The model under review builds one solid part; all positions refer to its coordinate system, in mm. A direction names the side the tool comes from. Round coordinates to 2 decimals unless told otherwise and drop trailing zeros. Write each loop counter-clockwise with the first axis right and the second up, starting at its lowest first coordinate (ties: lowest second). Pieces come first, ordered by that corner, then holes. Notation, with made-up numbers: M 66,49 L 85,49 A20 cw 85,83 Z; hole C 33,19.5 d8. An arc over 180 degrees is marked long. Write item = value, one per line. Start each with the question number.
Item 1: For pin 1 Ø3 at (y, z) = (16.02, 18.75) entering from +X; pin 2 Ø4 at (x, y) = (6, 7) entering from +Z; pin 3 Ø2 at (y, z) = (15, 16.5) entering from -X; pin 4 Ø7 at (x, z) = (10, 2) entering from +Y, all flat-tipped, find the tip position at first contact; note any pin that passes through.
Item 2: Take a section at D-D, the plane x = -10. Give the boundary of the cut face in (y, z), plus the area to 3 significant figures.
Item 3: Tool access review of faces 1 (the flat face through (7, -13.5, 2)), 2 (the flat face through (7, 13.5, 2)), 3 (the flat face through (0, 0, 3)): name each direction out of +Z, -Z, +X, -X, +Y, -Y from which nothing blocks a thin tool from reaching the whole face with its end or side.
Item 4: Take a section at A-A, the plane y = 0. Give the boundary of the cut face in (x, z), plus the area to 3 significant figures.
Item 5: To check wall thickness, follow line 1 along Y through (x, z) = (5, 2); line 2 along Y through (x, z) = (19.4, 18.75); line 3 along Z through (x, y) = (4.5, -4). State the ranges of each line that lie inside material, in increasing order.
Item 6: Take a section at C-C, the plane z = 28. Give the boundary of the cut face in (x, y).
Item 7: Take a section at B-B, the plane x = 5. Give the boundary of the cut face in (y, z).
Item 8: The part is to be moulded in two halves that separate along X. For faces 4 (the cylindrical face through (6.2, -8.04, 1.52)), 5 (the cylindrical face through (-11.789, -11.696, 1.521)), 6 (the cylindrical face through (19.02, 0.71, 49.99)), say which applies: +X half, -X half, draft (parallel to the pull), parting line (faces both ways), or undercut.
Autodesk Inventor part; units mm, degrees
ref_plane "YZ Plane" through (0, 0, 0) normal (1, 0, 0) x (0, 1, 0)
ref_plane "XZ Plane" through (0, 0, 0) normal (0, 1, 0) x (-1, 0, 0)
ref_plane "XY Plane" through (0, 0, 0) normal (0, 0, 1) x (1, 0, 0)
sketch "スケッチ1" plane through (0, 0, 0) normal (0, 0, 1) x (1, 0, 0)
  circle A0 centre (0, 0) radius 13.5
  line L0 (0, 13.5) -> (14.5, 13.5)
  line L1 (14.5, 13.5) -> (14.5, -13.5)
  line L2 (14.5, -13.5) -> (0, -13.5)
  line L3 (0, -13.5) -> (0, 13.5)
  line L4 (0, 0) -> (14.5, 0) construction
  point P0 (0, 13.5)
  point P1 (0, -13.5)
  point P2 (0, -13.5)
  dimension "d0" = 27
  dimension "d1" = 27
  dimension "d2" = 14.5
extrude "プレート1" add sketch "スケッチ1" along normal blind 3
sketch "スケッチ2" plane through (17.5, 13.5, 6) normal (1, 0, 0) x (0, 1, 0)
  line L0 (-27, 0) -> (0, 0)
  line L1 (0, 0) -> (0, 19)
  line L2 (0, 19) -> (-27, 19)
  line L3 (-27, 19) -> (-27, 0)
edge flange "フランジ1" height 25 angle 90 thickness 3 bend radius 3 thickness toward (1, 0, 0) relief tear relief width 3 relief depth 1.5 edges at (14.5, 0, 3) wall of the first edge with corners at (17.5, -13.5, 6) (17.5, 13.5, 6) (17.5, 13.5, 25) (17.5, -13.5, 25)
bend "曲げ1"
corner "コーナー1"
sketch "スケッチ3" plane through (0, 0, 0) normal (0, 0, -1) x (-1, 0, 0)
  point P0 (0, 0)
  point P1 (10, 0)
  point P2 (-5, 8.6603)
  point P3 (-5, -8.6603)
  dimension "d14" = 10
  dimension "d17" = 360
hole "穴1" at (-10, 0, 0) at (5, 8.6603, 0) at (5, -8.6603, 0) direction (0, 0, 1) diameter 2.7 depth 3
sketch "スケッチ4" plane through (20.5, -13.5, 25) normal (1, 0, 0) x (0, 0, -1)
  circle A0 centre (-3, 13.5) radius 22
  line L0 (25, 27) -> (25, 0)
  line L1 (0, 27) -> (19, 27)
  point P0 (25, 13.5)
  dimension "d26" = 44
  dimension "d29" = 28
  dimension "d46" = 13.5
extrude "押し出し1" add sketch "スケッチ4" against normal up to surface (3 mm away)
sketch "スケッチ5" plane through (20.5, -13.5, 6) normal (1, 0, 0) x (0, 0, -1)
  arc A0 (-4.629, 27) -> (-4.629, 0) centre (-22, 13.5) ccw
  circle A1 centre (-22, 13.5) radius 14.5
  point P0 (6, 13.5)
  dimension "d30" = 29
extrude "押し出し2" cut sketch "スケッチ5" against normal up to surface (3 mm away)
sketch "スケッチ6" plane through (20.5, 0, 28) normal (1, 0, 0) x (0, 0, 1)
  point P0 (-28, 0)
sketch "スケッチ7" plane through (20.5, -13.5, 6) normal (1, 0, 0) x (0, 0, -1)
  circle A0 centre (-22, 13.5) radius 14.5
  point P0 (6, 13.5)
  point P1 (-40.5, 13.5)
  point P2 (-12.75, -2.5215)
  point P3 (-12.75, 29.5215)
  dimension "d33" = 18.5
  dimension "d36" = 360
hole "穴2" at (20.5, 0, 46.5) at (20.5, -16.0215, 18.75) at (20.5, 16.0215, 18.75) direction (-1, 0, 0) diameter 2.7 depth 3
fillet "フィレット1" radius 10 2 edges at (19, -13.5, 10.629) (19, 13.5, 10.629)
sketch "スケッチ8" plane through (0, 0, 0) normal (0, 0, -1) x (-1, 0, 0)
  line L0 (0, 13.5) -> (-14.5, 13.5)
  line L1 (0, 13.5) -> (13.5, 13.5)
  line L2 (13.5, 13.5) -> (13.5, -13.5)
  line L3 (13.5, -13.5) -> (0, -13.5)
  line L4 (0, -13.5) -> (0, 13.5)
  circle A0 centre (-5, -8.6603) radius 1.35
  circle A1 centre (-5, 8.6603) radius 1.35
  circle A2 centre (10, 0) radius 1.35
  line L5 (0, 13.5) -> (-14.5, 13.5)
  line L6 (-14.5, 13.5) -> (-14.5, -13.5)
  line L7 (-14.5, -13.5) -> (0, -13.5)
  arc A3 (0, -13.5) -> (0, 13.5) centre (0, 0) ccw
  point P0 (13.5, 0)
  dimension "d47" = 13.5
  dimension "d48" = 27
extrude "押し出し3" add sketch "スケッチ8" against normal up to surface (3 mm away) contours L1 L2 A3 | A3 L2 L3
fillet "フィレット2" radius 6 2 edges at (-13.5, 13.5, 1.5) (-13.5, -13.5, 1.5)
equation "\"d24\" = Thickness"
equation "\"d3\" = Thickness"
equation "\"d4\" = BendReliefWidth"
equation "\"d5\" = BendReliefDepth"
equation "\"d6\" = MinimumRemnant"
equation "\"d7\" = TransitionRadius"
equation "\"d10\" = BendRadius"
equation "\"d11\" = CornerReliefSize"
equation "\"d12\" = GapSize"
equation "\"d13\" = JacobiRadiusSize"
equation "\"BendRadius\" = Thickness"
equation "\"BendReliefWidth\" = Thickness"
equation "\"BendReliefDepth\" = 0.5 * Thickness"
equation "\"CornerReliefSize\" = 4 * Thickness"
equation "\"MinimumRemnant\" = 2 * Thickness"
equation "\"TransitionRadius\" = BendRadius"
equation "\"JacobiRadiusSize\" = BendRadius"
equation "\"GapSize\" = Thickness"
properties part number "wrist_yaw_plate" material "アルミニウム 6061"
Response values:
q1.pin_1 = 20.5
q1.pin_2 = 3
q1.pin_3 = 17.5
q1.pin_4 = 13.5
q2.outline = M -12.95,0 L -1.35,0 L -1.35,3 L -12.95,3 Z; M 1.35,0 L 12.95,0 L 12.95,3 L 1.35,3 Z
q2.area = 69.6 mm2
q3.face_1 = -Z, +X, -X, -Y
q3.face_2 = -Z, +X, -X, +Y
q3.face_3 = +Z, -X, +Y, -Y
q4.outline = M -13.5,0 L -11.35,0 L -11.35,3 L -13.5,3 Z; M -8.65,0 L 14.5,0 A6 ccw 20.5,6 L 20.5,13.5 L 17.5,13.5 L 17.5,6 A3 cw 14.5,3 L -8.65,3 Z; M 17.5,42.5 L 20.5,42.5 L 20.5,45.15 L 17.5,45.15 Z; M 17.5,47.85 L 20.5,47.85 L 20.5,50 L 17.5,50 Z
q4.area = 134 mm2
q5.line_1 = -13.5 to -10.01, -7.31 to 7.31, 10.01 to 13.5
q5.line_2 = -19.96 to -17.37, -14.67 to -11.17, 11.17 to 14.67, 17.37 to 19.96
q5.line_3 = 0 to 3
q6.outline = M 17.5,-22 L 20.5,-22 L 20.5,-14.5 L 17.5,-14.5 Z; M 17.5,14.5 L 20.5,14.5 L 20.5,22 L 17.5,22 Z
q7.outline = M -13.5,0 L -10.01,0 L -10.01,3 L -13.5,3 Z; M -7.31,0 L 7.31,0 L 7.31,3 L -7.31,3 Z; M 10.01,0 L 13.5,0 L 13.5,3 L 10.01,3 Z
q8.face_4 = undercut
q8.face_5 = -X half
q8.face_6 = draft
